```python
from build123d import *

# Parameters (mm, degrees)
BOSS_EXTRUDE1_DEPTH = 25.4
SKETCH2_R           = 1.5875
CUT_EXTRUDE1_DEPTH  = 55.904554456
SPLIT1_DEPTH        = 25.4
SPLIT1_2_DEPTH      = 25.4


# Read off the part's stored shape, not the designer's step: Split1
with BuildPart() as part:
    # Sketch1 → Boss-Extrude1 (new body)
    with BuildSketch(Plane.XY):
        with BuildLine():
            Line((-10.795, 0), (10.795, 0))
            ThreePointArc((10.795, 0), (17.145, 6.35), (23.495, 0))
            Line((23.495, 0), (46.99, 0))
            Line((46.99, 0), (46.99, 3.175))
            Line((46.99, 3.175), (34.29, 3.175))
            Line((34.29, 3.175), (34.29, 15.875))
            Line((34.29, 15.875), (-34.29, 15.875))
            Line((-34.29, 15.875), (-34.29, 3.175))
            Line((-34.29, 3.175), (-46.99, 3.175))
            Line((-46.99, 3.175), (-46.99, 0))
            Line((-46.99, 0), (-23.495, 0))
            ThreePointArc((-23.495, 0), (-17.145, 6.35), (-10.795, 0))
        make_face()
    extrude(amount=BOSS_EXTRUDE1_DEPTH)

    # Sketch2 → Cut-Extrude1 (cut, through all)
    with BuildSketch(Plane(origin=(0, 3.175, 0), x_dir=(1, 0, 0), z_dir=(0, 1, 0))):
        with Locations(Location((40.64, -6.35, 0), (0, 0, 180))):
            Circle(SKETCH2_R)
        with Locations((40.64, -19.05)):
            Circle(SKETCH2_R)
        with Locations((-40.64, -6.35)):
            Circle(SKETCH2_R)
        with Locations(Location((-40.64, -19.05, 0), (0, 0, 180))):
            Circle(SKETCH2_R)
    extrude(amount=-CUT_EXTRUDE1_DEPTH, mode=Mode.SUBTRACT)

    # Split1 outline → Split1 (cut)
    with BuildSketch(Plane.XY):
        with BuildLine():
            add(Edge.make_bspline(
                [(34.29, 14.886313468), (26.866291946, 15.29633498), (15.604034158, 15.560800445), (0.522525145, 14.87798763), (-10.958660885, 13.761745583), (-22.480305747, 11.986676774), (-30.226096065, 10.175274204), (-34.155574129, 9.077862689), (-34.29, 9.040099193)],
                knots=[0.298916779, 0.298916779, 0.298916779, 0.298916779, 0.346600594, 0.371102737, 0.395726297, 0.420570145, 0.445825119, 0.446720069, 0.446720069, 0.446720069, 0.446720069], degree=3))
            Line((34.29, 14.886313468), (34.29, 15.875))
            Line((34.29, 15.875), (-34.29, 15.875))
            Line((-34.29, 15.875), (-34.29, 9.040099193))
        make_face()
    extrude(amount=SPLIT1_DEPTH, mode=Mode.SUBTRACT)


with BuildPart() as body_2:
    # Split1 2 outline → Split1 2 (new body)
    with BuildSketch(Plane.XY):
        with BuildLine():
            add(Edge.make_bspline(
                [(34.29, 14.886313468), (26.866291946, 15.29633498), (15.604034158, 15.560800445), (0.522525145, 14.87798763), (-10.958660885, 13.761745583), (-22.480305747, 11.986676774), (-30.226096065, 10.175274204), (-34.155574129, 9.077862689), (-34.29, 9.040099193)],
                knots=[0.298916779, 0.298916779, 0.298916779, 0.298916779, 0.346600594, 0.371102737, 0.395726297, 0.420570145, 0.445825119, 0.446720069, 0.446720069, 0.446720069, 0.446720069], degree=3))
            Line((34.29, 14.886313468), (34.29, 15.875))
            Line((34.29, 15.875), (-34.29, 15.875))
            Line((-34.29, 15.875), (-34.29, 9.040099193))
        make_face()
    extrude(amount=SPLIT1_2_DEPTH)


solid = part.part
```
Can you work these out from the model? Positions are in its coordinate system, mm. A direction names the side the tool comes from. Give positions to 0.01 mm unless a question says otherwise; leave off trailing zeros. Loops run counter-clockwise (first coordinate to the right, second up) from the corner with the lowest first, then second, coordinate; pieces in that order, holes last. Notation, with made-up numbers: M 83.25,57.5 L 90.25,57.5 A5 cw 90.25,63.5 Z; hole C 86,-36.75 d8. An arc over 180 degrees is marked long. Use one line per item in the form item = value. Start each with the question number.
(1) Thinking about a two-plate mould opening in X: for faces 1 (the cylindrical face through (17.01, 6.35, 12.52)), 2 (the flat face through (35, 0, 13)), 3 (the flat face through (34.29, 9, 13)), 4 (the flat face through (-46.99, 2, 13)), which applies, released by +X, released by -X, zero draft, split by the parting line, or undercut?
(2) Please list where these lines run through material, in increasing order: line 1 (Z direction, x = 40.64, y = 1.45); line 2 (X direction, y = 0.5, z = 17.25); line 3 (X direction, y = 2.5, z = 20.5).
(3) On a 3-axis mill with a long thin cutter (end or side, diameter ignored), from which of +Z, -Z, +X, -X, +Y, -Y can I reach the whole of each face in a straight line? I mean faces 5 (the flat face through (41, 3.175, 13)), 6 (the flat face through (46.99, 2, 13)), 7 (the flat face through (-41, 3.175, 13)). Say none if no direction works.
(4) I want a section at A-A, the plane x = 40.64. Write out the boundary of the cut face in (y, z) (1 decimal), and give its area (3 significant figures).
(5) I want a section at B-B, the plane z = 19.05. State how many separate pieces and enclosed holes the cut face has, and give its area (3 significant figures).
(6) I want a section at C-C, the plane y = 8.25. Write out the boundary of the cut face in (x, z), and give its area (3 significant figures).
(7) I'm going to push flat-ended pins straight in: P1, Ø3.5, axis at y = 9.5, z = 7.5, coming from the +X side; P2, Ø14, axis at x = -40.5, z = 6.5, coming from the +Y side; P3, Ø6.5, axis at x = 43, z = 17, coming from the +Y side (3 decimals). Where does each tip first touch, or does it pass through?
Worked out:
q1.face_1 = undercut
q1.face_2 = zero draft
q1.face_3 = released by +X
q1.face_4 = released by -X
q2.line_1 = 0 to 4.76, 7.94 to 17.46, 20.64 to 25.4
q2.line_2 = -46.99 to -23.48, -10.81 to 10.81, 23.48 to 46.99
q2.line_3 = -46.99 to -41.29, -39.99 to -22.98, -11.31 to 11.31, 22.98 to 39.99, 41.29 to 46.99
q3.face_5 = +Z, -Z, +X, +Y
q3.face_6 = +Z, -Z, +X, +Y, -Y
q3.face_7 = +Z, -Z, -X, +Y
q4.outline = M 0,0 L 3.2,0 L 3.2,4.8 L 0,4.8 Z; M 0,7.9 L 3.2,7.9 L 3.2,17.5 L 0,17.5 Z; M 0,20.6 L 3.2,20.6 L 3.2,25.4 L 0,25.4 Z
q4.area = 60.5 mm²
q5.separate_pieces = 3
q5.enclosed_holes = 0
q5.area = 882 mm²
q6.outline = M -34.29,0 L 34.29,0 L 34.29,25.4 L -34.29,25.4 Z
q6.area = 1,740 mm²
q7.P1 = 34.29
q7.P2 = 9.26
q7.P3 = 3.175
